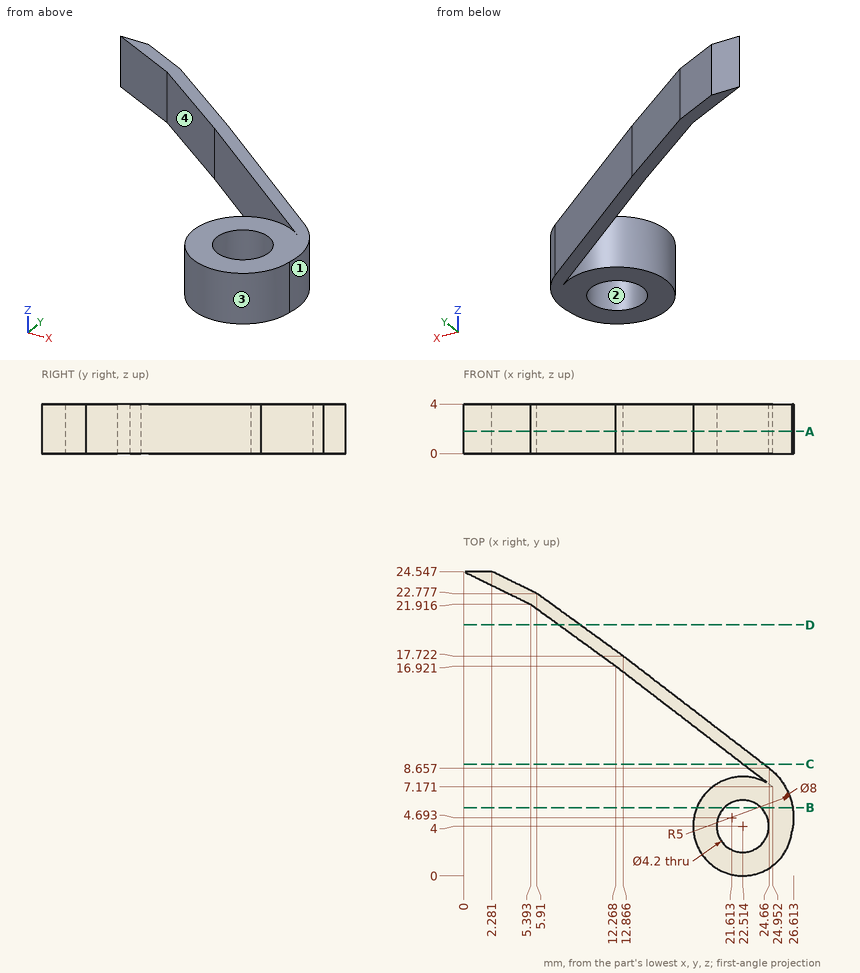
Study the drawing (mm; zero at the part's minimum x, y, z) and answer. Give positions to 0.01 mm unless a question says otherwise; leave off trailing zeros. Loops run counter-clockwise (first coordinate to the right, second up) from the corner with the lowest first, then second, coordinate; pieces in that order, holes last. Notation, with made-up numbers: (-35, 47.5) - (13, 47.5) arc R23 ccw to (13, 60.5) - close; hole circle Ø11 at (89, 3). An arc over 180 degrees is marked (long way). Use CSV: the item, a comma, the result in double quotes. Start each with the question number.
(1) Determine the mould class of the marked faces 1, 2, 3 and 4 for opening direction Y: released by +Y, released by -Y, zero draft, split by the parting line, or undercut.
(2) Each of these flat-tipped pins is pushed along its axis until it touches: pin 1 (3 mm diameter, centred on x = 18, y = 15.5, fed in from +Z); pin 2 (2 mm diameter, centred on y = 21.5, z = 3, fed in from +X) (1 decimal); pin 3 (1 mm diameter, centred on x = 21, z = 2.5, fed in from +Y) (1 decimal). Where does it stop, or does it pass through?
(3) Find section D-D, the plane y = 20.25. Determine the outline of the cut face in (x, z).
(4) Find section B-B, the plane y = 5.5. Determine the outline of the cut face in (x, z) (1 decimal).
(5) Find section C-C, the plane y = 9. Determine the outline of the cut face in (x, z).
(6) Find the intervals of material crossed by L1, parallel to Y at x = 23.25, z = 0.9 (1 decimal); L2, parallel to Y at x = 23, z = 1.2 (1 decimal); L3, parallel to X at y = 2.5, z = 1.35 (1 decimal), in increasing order.
(7) Find section A-A, the plane z = 1.8. Determine the outline of the cut face in (x, y) (1 decimal).
Results found:
1,face 1,"split by the parting line"
1,face 2,"undercut"
1,face 3,"undercut"
1,face 4,"released by -Y"
2,pin 1,"z = 4"
2,pin 2,"x = 9"
2,pin 3,"y = 11.9"
3,outline,"(7.69, 0) - (9.39, 0) - (9.39, 4) - (7.69, 4) - close"
4,outline,"(18.8, 0) - (21, 0) - (21, 4) - (18.8, 4) - close; (24, 0) - (26.5, 0) - (26.5, 4) - (24, 4) - close"
5,outline,"(22.57, 0) - (24.21, 0) - (24.21, 4) - (22.57, 4) - close"
6,L1,"0.1 to 2, 6 to 7.9, 8.5 to 9.7"
6,L2,"0 to 2, 6 to 8, 8.7 to 9.9"
6,L3,"18.8 to 21, 24 to 26.2"
7,outline,"(0, 24.5) - (5.4, 21.9) - (12.3, 16.9) - (25, 7.2) arc R4 ccw (long way) to (26.5, 3.6) arc R5 ccw to (24.7, 8.7) - (12.9, 17.7) - (5.9, 22.8) - (2.3, 24.5) - close; hole circle Ø4.2 at (22.5, 4)"
